Verification items for the finished model (mm, model axes). Round coordinates to 2 decimals unless told otherwise and drop trailing zeros. Order: outer loops, then holes, each group sorted by start corner. A loop starts at its lowest first (then second) coordinate and runs counter-clockwise, first axis right, second up. Notation, with made-up numbers: (21.5, 84.5) -> (51.5, 84.5) arc R32 ccw to (51.5, 111.5) -> close; hole circle Ø1 at (-25, 56.5). An arc over 180 degrees is marked (long way). Return JSON: item names as keys, results as strings. Group by question number.
Item 1: Depth check by flat-ended pin: pin 1 Ø4.5 at (x, y) = (0, 68.625) entering from -Z; pin 2 Ø1 at (x, y) = (-24.5, 63.5) entering from -Z. Enter the tip coordinate at first touch or a pass-through.
Item 2: Scan lines: probe 1 along Y at (x, z) = (0, 2) (3 decimals); probe 2 along Y at (x, z) = (-30, 4.5) (3 decimals); probe 3 along X at (y, z) = (-70, 5). Record each from-to range of solid material in increasing order. Write a range as from..to.
Item 3: Sectioned sample at A-A on x = 0. Record the cut outline in (y, z) (3 decimals).
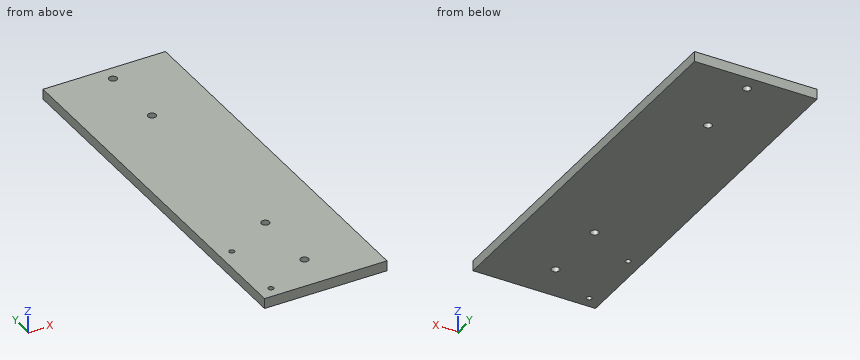
```python
from build123d import *

# Parameters (mm, degrees)
SKETCH1_W           = 76.2
SKETCH1_H           = 241.3
BOSS_EXTRUDE1_DEPTH = 6.35
M6_TAPPED_HOLE1_D   = 5
M4_TAPPED_HOLE1_D   = 3.3


with BuildPart() as part:
    # Sketch1 → Boss-Extrude1 (new body)
    with BuildSketch(Plane.XY):
        Rectangle(SKETCH1_W, SKETCH1_H)
    extrude(amount=BOSS_EXTRUDE1_DEPTH)

    # M6 Tapped Hole1 (through all)
    with Locations(Plane.XY.offset(6.35)):
        with Locations((0, -97.375), (0, 111.125), (0, -54.875), (0, 68.625)):
            Hole(M6_TAPPED_HOLE1_D / 2)

    # M4 Tapped Hole1 (through all)
    with Locations(Plane.XY.offset(6.35)):
        with Locations((-30, -70.875), (-30, -113.375)):
            Hole(M4_TAPPED_HOLE1_D / 2)


solid = part.part
```
Recorded:
{
 "1": {"pin 1": "through", "pin 2": "z = 0"},
 "2": {"probe 1": "-120.65..-99.875, -94.875..-57.375, -52.375..66.125, 71.125..108.625, 113.625..120.65", "probe 2": "-120.65..-115.025, -111.725..-72.525, -69.225..120.65", "probe 3": "-38.1..-31.4, -28.6..38.1"},
 "3": {"outline": "(-120.65, 0) -> (-99.875, 0) -> (-99.875, 6.35) -> (-120.65, 6.35) -> close; (-94.875, 0) -> (-57.375, 0) -> (-57.375, 6.35) -> (-94.875, 6.35) -> close; (-52.375, 0) -> (66.125, 0) -> (66.125, 6.35) -> (-52.375, 6.35) -> close; (71.125, 0) -> (108.625, 0) -> (108.625, 6.35) -> (71.125, 6.35) -> close; (113.625, 0) -> (120.65, 0) -> (120.65, 6.35) -> (113.625, 6.35) -> close"}
}
